Read the model definition and answer for the solid it produces. Units are mm, in the model's axes. A direction names the side the tool comes from. Give positions to 0.01 mm unless a question says otherwise; leave off trailing zeros. Write each loop counter-clockwise with the first axis right and the second up, starting at its lowest first coordinate (ties: lowest second). Pieces come first, ordered by that corner, then holes. Notation, with made-up numbers: (83.5, 1) -> (141.5, 1) arc R18 cw to (141.5, 34) -> close; hole circle Ø9 at (29.25, 38). An arc over 180 degrees is marked (long way). Write item = value, one per line.
Solid Edge part; units mm, degrees
sketch "Sketch1" plane through (0, 0, 0) normal (1, 0, 0) x (0, 1, 0)
  line L0 (0, -1.6764) -> (0, 1.6764)
  arc A0 (0, 1.6764) -> (5.55625, -1.6764) centre (-0.25374, -5.024398) cw
  line L1 (0, -1.6764) -> (5.55625, -1.6764)
revolve "RevolvedProtrusion1" add sketch "Sketch1" angle 360 about axis through (0, 0, -14.779625) along (0, 0, 1)
sketch "Sketch2" plane through (0, 0, -1.6764) normal (0, 0, -1) x (0, 1, 0)
  circle A0 centre (0, 0) radius 3.175
extrude "Protrusion1" add sketch "Sketch2" along normal blind 25.4
sketch "Sketch3" plane through (0, 0, -27.0764) normal (0, 0, -1) x (1, 0, 0)
  circle A0 centre (0, 0) radius 3.17246
extrude "Cutout1" cut sketch "Sketch3" against normal blind 23.8125 flip side to cut
sketch "Sketch4" plane through (-0.603226, 0.360624, 3.3528) normal (0, 0, 1) x (1, 0, 0)
  line L0 (-0.542454, 1.623751) -> (1.748905, 1.623751)
  line L1 (2.894585, -0.360624) -> (1.748905, 1.623751)
  line L2 (1.748905, -2.344999) -> (2.894585, -0.360624)
  line L3 (-0.542454, -2.344999) -> (1.748905, -2.344999)
  line L4 (-1.688133, -0.360624) -> (-0.542454, -2.344999)
  line L5 (-0.542454, 1.623751) -> (-1.688133, -0.360624)
extrude "ExtrudedCutout_11" cut sketch "Sketch4" against normal blind 5.0292
properties part number "24101086"
(1) The part is cut by section A-A on z = -24.5. Determine the outline of the cut face in (x, y), plus the area to 3 significant figures.
Checks:
outline = circle Ø6.34 at (0, 0)
area = 31.6 mm²
(2) A tool of negligible diameter and unlimited length cuts with its end or side. For faces 4 (the flat face through (1.727, 0.978, -0.169)), 5 (the flat face through (2.4, 2.4, -1.676)), from which of +Z, -Z, +X, -X, +Y, -Y can it reach the whole face along a straight path? Write none if from no direction.
Checks:
face_4 = +Z
face_5 = -Z
(3) For a pull along Y with two mould halves and no side action, classify faces 1 (the flat face through (0, 0, -27.076)), 2 (the flat face through (1.71, -1.01, -0.17)), 3 (the cylindrical face through (-0.413, -3.145, -15.337)) as released by +Y, released by -Y, zero draft, split by the parting line, or undercut.
Checks:
face_1 = zero draft
face_2 = undercut
face_3 = split by the parting line
(4) Consider L1, parallel to X at y = -0.5, z = -1; L2, parallel to Z at x = 1.25, y = 4; L3, parallel to Y at x = 0, z = -1. Determine where each line is inside the solid, lowest interval first.
Checks:
L1 = -5.09 to -2, 2 to 5.09
L2 = -1.68 to 0
L3 = -5.11 to -1.98, 1.98 to 5.11
(5) Given P1, Ø3, axis at x = -1, z = -10.5, coming from the +Y side; P2, Ø6, axis at x = 3.5, z = -2.5, coming from the +Y side; P3, Ø0.7, axis at x = 0, z = 0, coming from the -Y side, each flat-ended and moving along its own axis, determine where each tip first touches the part or whether it passes through.
Checks:
P1 = 3.17
P2 = 5.52
P3 = -4.55
